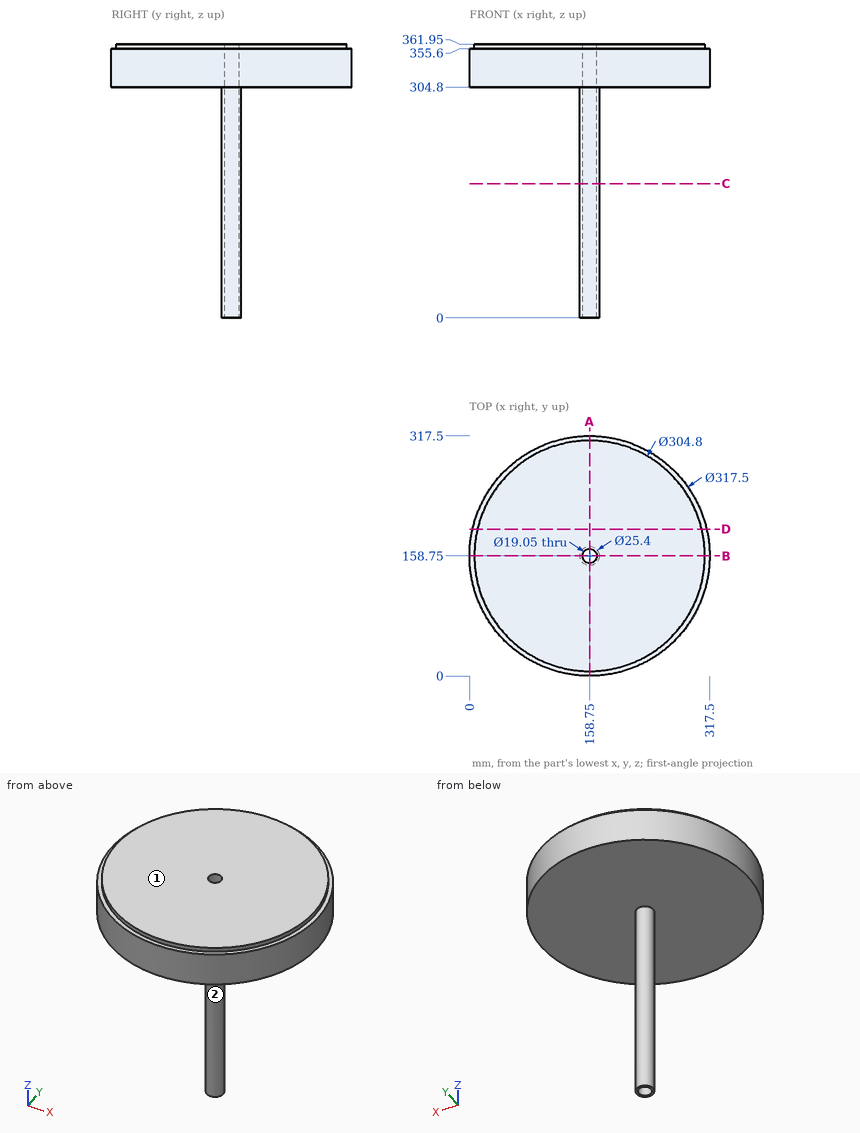
For this review, use the dimensioned drawing (mm, ordinates from the lowest corner) and the shaded views. A direction names the side the tool comes from. Give positions to 0.01 mm unless a question says otherwise; leave off trailing zeros. Write each loop counter-clockwise with the first axis right and the second up, starting at its lowest first coordinate (ties: lowest second). Pieces come first, ordered by that corner, then holes. Notation, with made-up numbers: M -1,64.25 L 56,64.25 A28 cw 56,95.25 Z; hole C 79,65 d4. An arc over 180 degrees is marked long. Write item = value, one per line. Start each with the question number.
Q1. We need section C-C (z = 177.5). State the section outline as (x, y) points (3 decimals).
Q2. We need section D-D (y = 194). State the section outline as (x, z) points, plus the area to 3 significant figures.
Q3. For line 1 (X direction, y = 158.75, z = 190.5) (3 decimals); line 2 (Z direction, x = 21, y = 100), list the stretches that pass through material, from the lowest coordinate up.
Q4. Machinability: for the marked faces 1 and 2, which of the approach directions +Z, -Z, +X, -X, +Y, -Y give a long, thin tool a straight path to every point of the face, cutting with its end or side? Answer none if there is none.
Q5. We need section A-A (x = 158.75). State the section outline as (y, z) points (3 decimals), plus the area to 3 significant figures.
Q6. Clearance check with flat-ended pins moving along their axes: pin 1 (6 mm diameter, centred on y = 175.5, z = 237, fed in from +X); pin 2 (5 mm diameter, centred on x = 115, y = 87, fed in from -Z). State where each tip first meets the part, or that it passes through.
Result set:
q1.outline = C 158.75,158.75 d25.4; hole C 158.75,158.75 d19.05
q2.outline = M 3.96,304.8 L 313.54,304.8 L 313.54,355.6 L 307.02,355.6 L 307.02,361.95 L 10.48,361.95 L 10.48,355.6 L 3.96,355.6 Z
q2.area = 17,600 mm2
q3.line_1 = 146.05 to 149.225, 168.275 to 171.45
q3.line_2 = 304.8 to 361.95
q4.face_1 = +Z, +X, -X, +Y, -Y
q4.face_2 = -Z
q5.outline = M 0,304.8 L 146.05,304.8 L 146.05,0 L 149.225,0 L 149.225,361.95 L 6.35,361.95 L 6.35,355.6 L 0,355.6 Z; M 168.275,0 L 171.45,0 L 171.45,304.8 L 317.5,304.8 L 317.5,355.6 L 311.15,355.6 L 311.15,361.95 L 168.275,361.95 Z
q5.area = 18,900 mm2
q6.pin_1 = through
q6.pin_2 = 304.8
